Check sheet for the modelled part. Datum: model origin and axes. Units: mm. A direction names the side the tool comes from. Round coordinates to 2 decimals unless told otherwise and drop trailing zeros. Loops run counter-clockwise (first coordinate to the right, second up) from the corner with the lowest first, then second, coordinate; pieces in that order, holes last. Notation, with made-up numbers: (0, 66) - (30, 66) arc R25 ccw to (30, 97) - close; hole circle Ø3 at (-0.75, 21). An arc over 180 degrees is marked (long way). Put each result on its own line as item: value. Start each with the question number.
Item 1: Section check C-C, the plane x = 14. Record the cut outline in (y, z), and give its area (3 significant figures).
Item 2: Section check B-B, the plane y = 12. Record the cut outline in (x, z), and give its area (3 significant figures).
Item 3: Draft check along X on faces 1 (the flat face through (0, 5, 1)), 2 (the flat face through (40.239, -3, 1)), 3 (the flat face through (49.087, 20.817, 1.479)). Enter one of: pulls with the +X half, pulls with the -X half, needs draft (parallel to the pull), parting line crosses it, or undercut.
Item 4: Tool access check on faces 4 (the flat face through (3, -1, 1)), 5 (the flat face through (37, -1.499, 1)), 6 (the flat face through (52, 10, 1)). Record the directions out of +Z, -Z, +X, -X, +Y, -Y that give a thin tool (end or side, any length) a straight path to the whole face; none if there is none.
Item 5: Material ranges on line 1 along X through (y, z) = (25, 1.85); line 2 along Y through (x, z) = (20.5, 0.8); line 3 along Y through (x, z) = (42, 1.85), recorded low to high.
Item 6: Gauge pin test, flat ends, axial feed: pin 1 Ø1.5 at (y, z) = (11.5, 1) entering from -X; pin 2 Ø1.5 at (x, z) = (2, 2) entering from +Y; pin 3 Ø1.5 at (x, z) = (2, 2) entering from -Y; pin 4 Ø2 at (x, y) = (22, 21.5) entering from +Z. Record the tip position at first contact, or that the pin passes through.
from build123d import *

# Parameters (mm, degrees)
SKETCH_1_R      = 1.35
EXTRUDE_1_DEPTH = 3


with BuildPart() as part:
    # 草图1 → 凸台-拉伸1 (new body)
    with BuildSketch(Plane(origin=(0, 0, 0), x_dir=(-1, 0, 0), z_dir=(0, 0, -1))):
        with BuildLine():
            Line((-41.246222879, 31.4756), (-41.70566582, 31.4756))
            ThreePointArc((-41.70566582, 31.4756), (-45.386541118, 30.213865193), (-47.519320255, 26.959319012))
            Line((-47.519320255, 26.959319012), (-50.6992, 14.4996))
            Line((-50.6992, 14.4996), (-50.6992, 10.0003))
            Line((-50.6992, 10.0003), (-53.6992, 10.0003))
            Line((-53.6992, 10.0003), (-53.6992, 0))
            Line((-53.6992, 0), (-50.6992, 0))
            Line((-50.6992, 0), (-50.6992, -1.5007))
            Line((-50.6992, -1.5007), (-49.2382, -1.5007))
            Line((-49.2382, -1.5007), (-49.2382, -4.5007))
            Line((-49.2382, -4.5007), (-40.2392, -4.5007))
            Line((-40.2392, -4.5007), (-40.2392, -1.4993))
            Line((-40.2392, -1.4993), (-34.2002, -1.4993))
            Line((-34.2002, -1.4993), (-34.2002, 1.0005))
            Line((-34.2002, 1.0005), (-19.2003, 1.0005))
            Line((-19.2003, 1.0005), (-19.2003, -1.4993))
            Line((-19.2003, -1.4993), (-11.7217, -1.4993))
            Line((-11.7217, -1.4993), (-11.7217, -4.5007))
            Line((-11.7217, -4.5007), (-4.3215, -4.5007))
            Line((-4.3215, -4.5007), (-4.3215, -1.5007))
            Line((-4.3215, -1.5007), (-3, -1.5007))
            Line((-3, -1.5007), (-3, 0))
            Line((-3, 0), (0, 0))
            Line((0, 0), (0, 10.0003))
            Line((0, 10.0003), (-3, 10.0003))
            Line((-3, 10.0003), (-3, 14.4996))
            Line((-3, 14.4996), (-26.543543046, 20.807804388))
            ThreePointArc((-26.543543046, 20.807804388), (-32.65852857, 22.990550509), (-36.548909006, 28.188854909))
            ThreePointArc((-36.548909006, 28.188854909), (-38.379715818, 30.572322748), (-41.246222879, 31.4756))
        make_face()
        with Locations((-41.6992, 25.49975)):
            Circle(SKETCH_1_R, mode=Mode.SUBTRACT)
    extrude(amount=-EXTRUDE_1_DEPTH)


solid = part.part
Check result:
1. outline: (-1.5, 0) - (17.45, 0) - (17.45, 3) - (-1.5, 3) - close
1. area: 56.8 mm²
2. outline: (3, 0) - (50.7, 0) - (50.7, 3) - (3, 3) - close
2. area: 143 mm²
3. face 1: pulls with the -X half
3. face 2: undercut
3. face 3: pulls with the +X half
4. face 4: +Z, -Z, -X, -Y
4. face 5: +Z, -Z, -Y
4. face 6: +Z, -Z, +X, +Y
5. line 1: 34.75 to 40.45, 42.95 to 48.02
5. line 2: 1 to 19.19
5. line 3: -4.5 to 24.18, 26.82 to 31.47
6. pin 1: x = 3
6. pin 2: y = 10
6. pin 3: y = 0
6. pin 4: through
